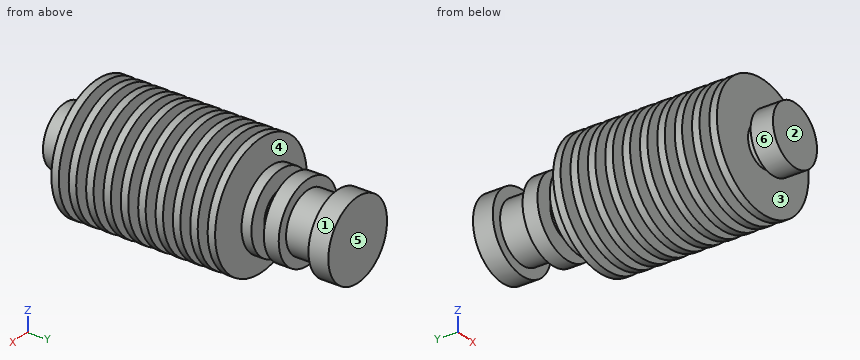
```python
from build123d import *


with BuildPart() as part:
    # Sketch1 → Revolve1 (revolve)
    with BuildSketch(Plane.XY):
        Polygon((0, 29.5), (8, 29.5), (8, 25.5), (6, 25.5), (6, 19.5), (8, 19.5), (8, 16.5), (4.5, 16.5), (4.5, 14), (8, 14), (8, 12), (4.5, 12), (4.5, 10), (12.5, 10), (12.5, 8.5), (4.5, 8.5), (4.5, 6.5), (12.5, 6.5), (12.5, 5), (4.5, 5), (4.5, 3), (12.5, 3), (12.5, 1.5), (4.5, 1.5), (4.5, -0.5), (12.5, -0.5), (12.5, -2), (6.5, -2), (6.5, -4), (12.5, -4), (12.5, -5.5), (7.5, -5.5), (7.5, -7.5), (12.5, -7.5), (12.5, -9), (7.5, -9), (7.5, -11), (12.5, -11), (12.5, -12.5), (7.5, -12.5), (7.5, -14.5), (12.5, -14.5), (12.5, -16), (7.5, -16), (7.5, -18), (12.5, -18), (12.5, -19.5), (7.5, -19.5), (7.5, -21.5), (12.5, -21.5), (12.5, -23), (4, -23), (4, -25), (6, -25), (6, -29.5), (0, -29.5), align=None)
    revolve(axis=Axis((0, -29.5, 0), (0, 1, 0)))


solid = part.part
```
Check sheet for the modelled part. Datum: model origin and axes. Units: mm. Face numbers are marked on the shaded views. A direction names the side the tool comes from. Give positions to 0.01 mm unless a question says otherwise; leave off trailing zeros. Write each loop counter-clockwise with the first axis right and the second up, starting at its lowest first coordinate (ties: lowest second). Pieces come first, ordered by that corner, then holes. Notation, with made-up numbers: (45.5, 83) - (104.5, 83) arc R26 cw to (104.5, 121) - close; hole circle Ø8 at (88, 21.5). An arc over 180 degrees is marked (long way). Answer as a JSON object with one key per item and string values. Group by question number.
1) Access from +Z, -Z, +X, -X, +Y, -Y to the whole of each face (thin tool, end or side, straight path). Record for the marked faces 1, 2 and 3.
2) Thickness scan on probe 1 along Y at (x, z) = (-3.75, 1.5); probe 2 along Z at (x, y) = (0.25, -27); probe 3 along Z at (x, y) = (-3.25, -4.5). Record the ranges inside material, lowest first. Write a range as from..to.
3) Release check for a two-part mould opening along Y. For the marked faces 4, 5 and 6 record: pulls with the +Y half, pulls with the -Y half, needs draft (parallel to the pull), parting line crosses it, or undercut.
4) Sectioned sample at B-B (y = 23). Record the cut outline in (x, z).
5) Sectioned sample at A-A (z = -10). Give the number of separate pieces and of enclosed holes in the cut face, then the cut area to 3 significant figures.
6) Depth check by flat-ended pin: P1, Ø5, axis at y = 20, z = 9.5, coming from the +X side; P2, Ø10, axis at y = -7.5, z = -6.5, coming from the +X side; P3, Ø2, axis at x = -5.5, z = -9.5, coming from the +Y side. Enter the tip coordinate at first touch or a pass-through.
Geometry results:
{
 "1": {"face 1": "+Y", "face 2": "+Z, -Z, +X, -X, -Y", "face 3": "none"},
 "2": {"probe 1": "y = -29.5..-25, -23..29.5", "probe 2": "z = -5.99..5.99", "probe 3": "z = -12.07..12.07"},
 "3": {"face 4": "undercut", "face 5": "pulls with the +Y half", "face 6": "needs draft"},
 "4": {"outline": "circle Ø12 at (0, 0)"},
 "5": {"separate pieces": "10", "enclosed holes": "0", "area": "225 mm^2"},
 "6": {"P1": "stops at x = 3.78", "P2": "stops at x = 12.41", "P3": "stops at y = 10"}
}
